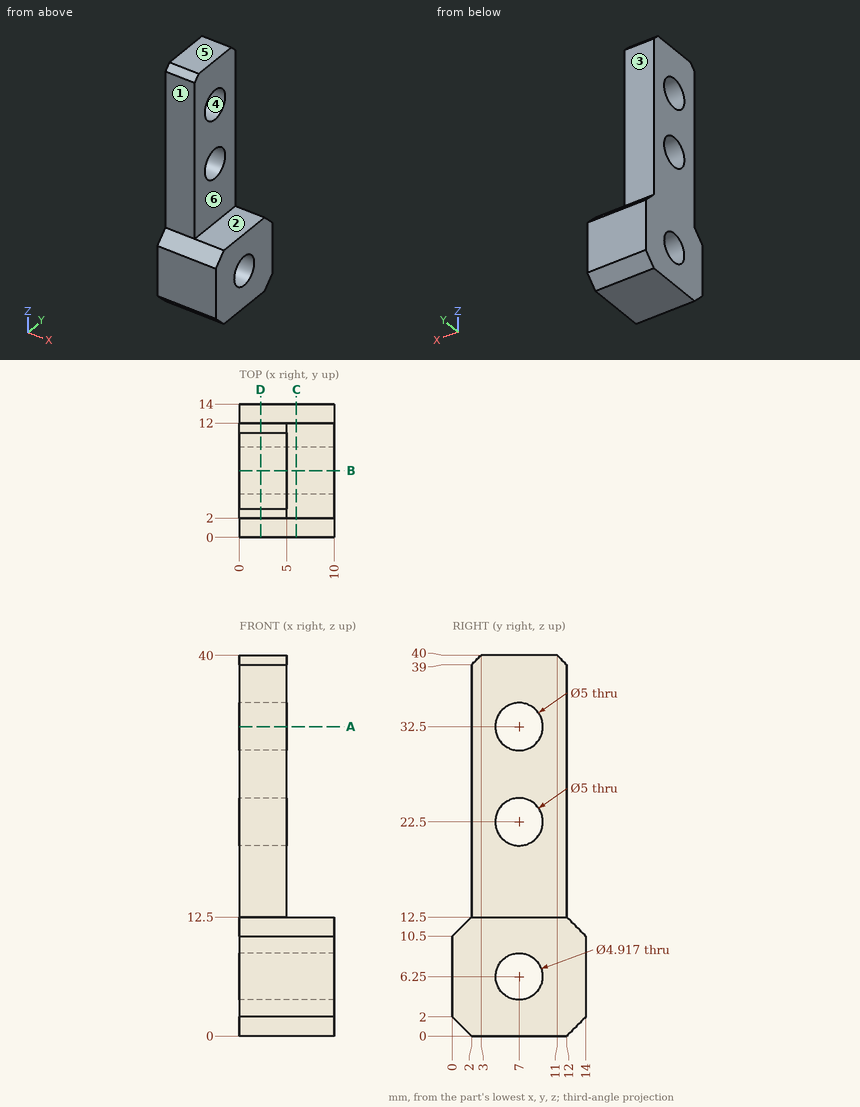
The figure shows three views and two pictorial views of one solid part (mm, origin at its lowest corner). Answer the questions. A direction names the side the tool comes from. Give positions to 0.01 mm unless a question says otherwise; leave off trailing zeros. Write each loop counter-clockwise with the first axis right and the second up, starting at its lowest first coordinate (ties: lowest second). Pieces come first, ordered by that corner, then holes.
Q1. A tool of negligible diameter and unlimited length cuts with its end or side. For the marked faces 1, 2 and 3, from which of +Z, -Z, +X, -X, +Y, -Y can it reach the whole face along a straight path? Write none if from no direction.
Answer:
face 1: +Z, +X, -X, -Y
face 2: +Z, +X, +Y, -Y
face 3: +Z, +X, -X, +Y
Q2. The part is cut by section B-B on y = 7. Give the vertices of the cut face in (x, z).
Answer:
outline: (0, 0) - (10, 0) - (10, 3.79) - (0, 3.79) - close; (0, 8.71) - (10, 8.71) - (10, 12.5) - (5, 12.5) - (5, 20) - (0, 20) - close; (0, 25) - (5, 25) - (5, 30) - (0, 30) - close; (0, 35) - (5, 35) - (5, 40) - (0, 40) - close
Q3. Straight lines are drawn through the part: L1, parallel to Y at x = 7, z = 6.25; L2, parallel to Z at x = 4, y = 6; L3, parallel to Y at x = 2, z = 30.5. For each, find the intervals that lie inside material, in ascending order.
Answer:
L1: y = 0 to 4.54, 9.46 to 14
L2: z = 0 to 4, 8.5 to 20.21, 24.79 to 30.21, 34.79 to 40
L3: y = 2 to 5.5, 8.5 to 12
Q4. The part is cut by section A-A on z = 32.5. Give the vertices of the cut face in (x, y).
Answer:
outline: (0, 2) - (5, 2) - (5, 4.5) - (0, 4.5) - close; (0, 9.5) - (5, 9.5) - (5, 12) - (0, 12) - close
Q5. The part is cut by section D-D on x = 2.25. Give the vertices of the cut face in (y, z).
Answer:
outline: (0, 2) - (2, 0) - (12, 0) - (14, 2) - (14, 10.5) - (12, 12.5) - (12, 39) - (11, 40) - (3, 40) - (2, 39) - (2, 12.5) - (0, 10.5) - close; hole circle Ø5 at (7, 22.5); hole circle Ø5 at (7, 32.5); hole circle Ø4.92 at (7, 6.25)
Q6. The part is cut by section C-C on x = 6. Give the vertices of the cut face in (y, z).
Answer:
outline: (0, 2) - (2, 0) - (12, 0) - (14, 2) - (14, 10.5) - (12, 12.5) - (2, 12.5) - (0, 10.5) - close; hole circle Ø4.92 at (7, 6.25)
Q7. Given pin 1 (4 mm diameter, centred on x = 8.5, y = 6, fed in from +Z); pin 2 (1 mm diameter, centred on y = 4.5, z = 33.5, fed in from +X); pin 3 (3 mm diameter, centred on x = 4.5, z = 32.5, fed in from +Y); pin 4 (4 mm diameter, centred on y = 7, z = 22.5, fed in from -X), each flat-ended and moving along its own axis, determine where each tip first touches the part or whether it passes through.
Answer:
pin 1: stops at z = 12.5
pin 2: stops at x = 5
pin 3: stops at y = 12
pin 4: passes through
Q8. For a pull along Z with two mould halves and no side action, classify the marked faces 4, 5 and 6 as released by +Z, released by -Z, zero draft, split by the parting line, or undercut.
Answer:
face 4: undercut
face 5: released by +Z
face 6: zero draft
